```python
from build123d import *


with BuildPart() as f1:
    # F0 (on Top) → F1 (revolve)
    with BuildSketch(Plane.XY):
        with BuildLine():
            Line((32.2443948891, 40.8806465566), (0, 40.8806465566))
            Line((0, 40.8806465566), (0, -7.8476248309))
            Line((0, -7.8476248309), (23.1651897523, -7.8476248309))
            ThreePointArc((23.1651897523, -7.8476248309), (23.2494349236, -9.7712701453), (23.5015253586, -11.6801857948))
            Line((23.5015253586, -11.6801857948), (0, -11.6801857948))
            Line((0, -11.6801857948), (0, -43.4356927872))
            Line((0, -43.4356927872), (65.6097978354, -43.4356927872))
            Line((65.6097978354, -43.4356927872), (65.6097978354, -15.9950943577))
            ThreePointArc((65.6097978354, -15.9950943577), (63.3830284541, 4.4996240423), (45.1694689691, 14.1566543859))
            Line((45.1694689691, 14.1566543859), (45.1694689691, 27.1900529973))
            add(Edge.make_bspline(
                [(45.1694689691, 27.1900529973), (64.1933435471, 21.4488804325), (61.7417399221, 46.9721411104), (59.2901362971, 72.4954017883), (41.1770152264, 68.7548624879), (23.0638941557, 65.0143231875), (32.2443948891, 40.8806465566)],
                knots=[5.8712915917, 5.8712915917, 5.8712915917, 7.6289194311, 7.6289194311, 9.3865472704, 9.3865472704, 11.1441751097, 11.1441751097, 11.1441751097], degree=2, weights=[1, 0.638064854, 1, 0.638064854, 1, 0.638064854, 1]))
        make_face()
    revolve(axis=Axis((0, 0.4562586546, 0), (0, -1, 0)))


solid = f1.part
```
Part model, mm, in its own coordinate system. Coordinates: 2 decimals unless noted, no trailing zeros. Write each loop counter-clockwise with the first axis right and the second up, starting at its lowest first coordinate (ties: lowest second). Pieces come first, ordered by that corner, then holes.
Item 1: Mould opens along Z. For faces 1 (the face through (0, -11.68, 0)), 2 (the face through (-14.22, -29.52, -64.05)), 3 (the face through (1, -43.436, 1)) say: released by +Z, released by -Z, zero draft, split by the parting line, or undercut.
Item 2: Probe line 1 (Y direction, x = 15, z = 15); line 2 (Z direction, x = 24, y = 52.5); line 3 (Y direction, x = -19, z = 42). List the from-to ranges inside material, lowest first.
Item 3: Pin check, flat tips, straight feed: pin 1 (1 mm diameter, centred on x = 15, y = 52.5, fed in from +Z); pin 2 (1 mm diameter, centred on y = -3.5, z = 47.5, fed in from +X); pin 3 (3 mm diameter, centred on y = 23.5, z = 23, fed in from -X). Stop position of each tip, or through.
Item 4: Slice it at B-B (y = 22). Write the cut outline in (x, z).
Item 5: Slice it at A-A (y = -36). Write the cut outline in (x, z).
Results found:
1. face 1: undercut
1. face 2: split by the parting line
1. face 3: zero draft
2. line 1: y = -43.44 to -11.68, -7.85 to 40.88
2. line 2: z = -55.73 to -18.52, 18.52 to 55.73
2. line 3: y = -43.44 to 14.14, 26.95 to 68.68
3. pin 1: stops at z = 58.99
3. pin 2: stops at x = 47.4
3. pin 3: stops at x = -39.72
4. outline: circle Ø90.34 at (0, 0)
5. outline: circle Ø131.22 at (0, 0)
